Check sheet for the modelled part. Datum: model origin and axes. Units: mm. Round coordinates to 2 decimals unless told otherwise and drop trailing zeros. Order: outer loops, then holes, each group sorted by start corner. A loop starts at its lowest first (then second) coordinate and runs counter-clockwise, first axis right, second up.
Q1. Cross-section at B-B on y = 15. Record the cut outline in (x, z), then the cut area to 3 significant figures.
Q2. Cross-section at C-C on z = -20. Record the cut outline in (x, y), then the cut area to 3 significant figures.
Q3. Scan lines: probe 1 along Z at (x, y) = (0.6, 6.5); probe 2 along Y at (x, z) = (0.5, 8); probe 3 along Z at (x, y) = (0.3, 15.5). Record each from-to range of solid material in increasing order.
Q4. Cross-section at D-D on x = 0.65. Record the cut outline in (y, z), then the cut area to 3 significant figures.
Q5. Cross-section at A-A on z = 11.5. Record the cut outline in (x, y), then the cut area to 3 significant figures.
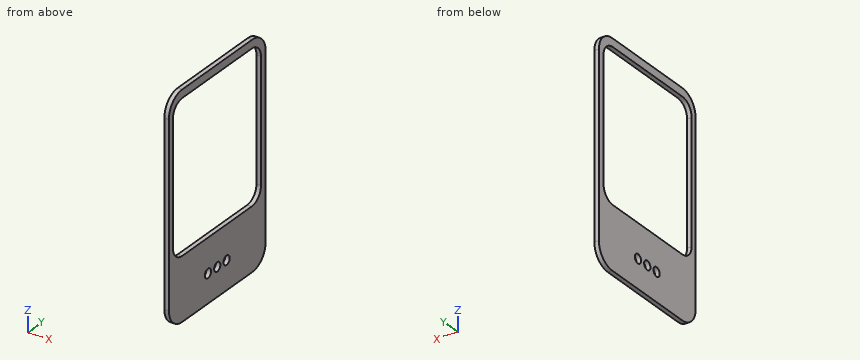
from build123d import *

# Parameters (mm, degrees)
EXTRUDE_1_DEPTH     = 1
CUT_EXTRUDE_1_DEPTH = 2
SKETCH_3_R          = 1
CUT_EXTRUDE_2_DEPTH = 2


with BuildPart() as part:
    # 草图1 → 凸台-拉伸1 (new body)
    with BuildSketch(Plane(origin=(0, 0, 0), x_dir=(0, 0, -1), z_dir=(1, 0, 0))):
        with BuildLine():
            Line((26.809806157, -1.747534601), (26.809806157, 20.752465399))
            ThreePointArc((26.809806157, 20.752465399), (25.550365316, 23.793024558), (22.509806157, 25.052465399))
            Line((22.509806157, 25.052465399), (-17.490193843, 25.052465399))
            ThreePointArc((-17.490193843, 25.052465399), (-20.530753002, 23.793024558), (-21.790193843, 20.752465399))
            Line((-21.790193843, 20.752465399), (-21.790193843, -1.747534601))
            ThreePointArc((-21.790193843, -1.747534601), (-20.530753002, -4.78809376), (-17.490193843, -6.047534601))
            Line((-17.490193843, -6.047534601), (22.509806157, -6.047534601))
            ThreePointArc((22.509806157, -6.047534601), (25.550365316, -4.78809376), (26.809806157, -1.747534601))
        make_face()
    extrude(amount=EXTRUDE_1_DEPTH)

    # 草图2 → 切除-拉伸1 (cut, through all)
    with BuildSketch(Plane.ZY):
        with BuildLine():
            Line((-13.009806157, 20.552465399), (-13.009806157, -1.747534601))
            ThreePointArc((-13.009806157, -1.747534601), (-12.131126501, -3.868854944), (-10.009806157, -4.747534601))
            Line((-10.009806157, -4.747534601), (16.990193843, -4.747534601))
            ThreePointArc((16.990193843, -4.747534601), (19.111514186, -3.868854944), (19.990193843, -1.747534601))
            Line((19.990193843, -1.747534601), (19.990193843, 20.552465399))
            ThreePointArc((19.990193843, 20.552465399), (19.111514186, 22.673785743), (16.990193843, 23.552465399))
            Line((16.990193843, 23.552465399), (-10.009806157, 23.552465399))
            ThreePointArc((-10.009806157, 23.552465399), (-12.131126501, 22.673785743), (-13.009806157, 20.552465399))
        make_face()
    extrude(amount=-CUT_EXTRUDE_1_DEPTH, mode=Mode.SUBTRACT)

    # 草图3 → 切除-拉伸2 (cut, through all)
    with BuildSketch(Plane.ZY):
        with Locations((-20.491320576, 6.494332556)):
            Circle(SKETCH_3_R)
        with Locations((-20.509806157, 9.502465399)):
            Circle(SKETCH_3_R)
        with Locations((-20.509806157, 12.502465399)):
            Circle(SKETCH_3_R)
    extrude(amount=-CUT_EXTRUDE_2_DEPTH, mode=Mode.SUBTRACT)


solid = part.part
Results found:
1. outline: (0, -26.81) - (1, -26.81) - (1, -13.01) - (0, -13.01) - close; (0, 19.99) - (1, 19.99) - (1, 21.79) - (0, 21.79) - close
1. area: 15.6 mm2
2. outline: (0, -6.05) - (1, -6.05) - (1, 5.62) - (0, 5.62) - close; (0, 7.37) - (1, 7.37) - (1, 8.64) - (0, 8.64) - close; (0, 10.36) - (1, 10.36) - (1, 11.64) - (0, 11.64) - close; (0, 13.36) - (1, 13.36) - (1, 25.05) - (0, 25.05) - close
2. area: 25.9 mm2
3. probe 1: z = -26.81 to -21.49, -19.49 to -13.01, 19.99 to 21.79
3. probe 2: y = -6.05 to -4.75, 23.55 to 25.05
3. probe 3: z = -26.81 to -13.01, 19.99 to 21.79
4. outline: (-6.05, -22.51) arc R4.3 ccw to (-1.75, -26.81) - (20.75, -26.81) arc R4.3 ccw to (25.05, -22.51) - (25.05, 17.49) arc R4.3 ccw to (20.75, 21.79) - (-1.75, 21.79) arc R4.3 ccw to (-6.05, 17.49) - close; hole (-4.75, -10.01) arc R3 ccw to (-1.75, -13.01) - (20.55, -13.01) arc R3 ccw to (23.55, -10.01) - (23.55, 16.99) arc R3 ccw to (20.55, 19.99) - (-1.75, 19.99) arc R3 ccw to (-4.75, 16.99) - close; hole circle Ø2 at (6.49, -20.49); hole circle Ø2 at (9.5, -20.51); hole circle Ø2 at (12.5, -20.51)
4. area: 560 mm2
5. outline: (0, -6.05) - (1, -6.05) - (1, -4.75) - (0, -4.75) - close; (0, 23.55) - (1, 23.55) - (1, 25.05) - (0, 25.05) - close
5. area: 2.80 mm2
